Geometry: final body of the model. Coordinates: model frame, mm. A direction names the side the tool comes from. Give positions to 0.01 mm unless a question says otherwise; leave off trailing zeros. Order: outer loops, then holes, each group sorted by start corner. A loop starts at its lowest first (then second) coordinate and runs counter-clockwise, first axis right, second up. Notation, with made-up numbers: (-23, 29) -> (14, 29) arc R11 ccw to (14, 43) -> close; hole circle Ø4 at (-29.5, 28). An arc over 180 degrees is marked (long way). One line per question, with ' | ' between items. Start each with the question number.
(1) Mould query, pull axis X, two halves, no side actions, for faces 1 (the face through (29.083, 8, 11)), 2 (the face through (-38.1, 7, 0)), 3 (the face through (-1, 0, 0)). Classes: +X half, -X half, draft (parallel to the pull), parting line (faces both ways), or undercut.
(2) Section C-C (z = 0). Return loops of the section in (x, y).
(3) Section D-D (z = 19.05). Return loops of the section in (x, y).
(4) Ray query, L1, parallel to Z at x = 0, y = 10; L2, parallel to X at y = 7, z = -19.05; L3, parallel to Z at x = 31.75, y = 4.75. Return the intervals inside material, ascending.
(5) First-contact query: pin 1 Ø3 at (x, z) = (0, -19.05) entering from -Y; pin 2 Ø10 at (x, z) = (-13, -7) entering from +Y. Flat tips, straight axial feed; report the tip coordinate or a pass-through.
(6) Section A-A (x = -31.75). Return loops of the section in (y, z), then the cut area to 3 significant figures.
(7) Section B-B (x = 0). Return loops of the section in (y, z), then the cut area to 3 significant figures.
(8) Set-up query: faces 4 (the face through (33.676, 6.439, -0.607)), 5 (the face through (28.105, 7.879, -7.381)). Return all of +Z, -Z, +X, -X, +Y, -Y with unobstructed straight access to the full face (end or side cutting, diameter ignored); none if empty.
```python
from build123d import *

# Parameters (mm, degrees)
SKETCH1_W              = 76.2
SKETCH1_H              = 50.8
BOSS_EXTRUDE1_DEPTH    = 12.7
SKETCH2_W              = 51.308
SKETCH2_H              = 25.908
CUT_EXTRUDE1_DEPTH     = 9.779
CUT_EXTRUDE2_DEPTH     = 9.779
MIRROR2_COPY_1_DEPTH   = 9.779
F_10_32_TAPPED_HOLE1_D = 4.0386
CHAMFER1_SIZE          = 3.175
FILLET1_R              = 0.508
CHAMFER2_SIZE          = 0.508
F_10_32_TAPPED_HOLE2_D = 4.0386


with BuildPart() as part:
    # Sketch1 → Boss-Extrude1 (new body)
    with BuildSketch(Plane(origin=(0, 0, 0), x_dir=(1, 0, 0), z_dir=(0, 1, 0))):
        Rectangle(SKETCH1_W, SKETCH1_H)
    extrude(amount=BOSS_EXTRUDE1_DEPTH)

    # Sketch2 → Cut-Extrude1 (cut)
    with BuildSketch(Plane(origin=(0, 12.7, 0), x_dir=(1, 0, 0), z_dir=(0, 1, 0))):
        Rectangle(SKETCH2_W, SKETCH2_H)
    extrude(amount=-CUT_EXTRUDE1_DEPTH, mode=Mode.SUBTRACT)

    # Sketch3 → Cut-Extrude2 (cut)
    with BuildSketch(Plane(origin=(0, 12.7, 0), x_dir=(1, 0, 0), z_dir=(0, 1, 0))):
        with BuildLine():
            Line((-22.479, 16.383), (-25.654, 16.383))
            ThreePointArc((-25.654, 16.383), (-28.078669153, 15.378669153), (-29.083, 12.954))
            Line((-29.083, 12.954), (-29.083, 9.779))
            ThreePointArc((-29.083, 9.779), (-26.96622149, 6.611017083), (-23.229330847, 7.354330847))
            Line((-23.229330847, 7.354330847), (-20.054330847, 10.529330847))
            ThreePointArc((-20.054330847, 10.529330847), (-19.311017083, 14.26622149), (-22.479, 16.383))
        make_face()
    cut_extrude2 = extrude(amount=-CUT_EXTRUDE2_DEPTH, mode=Mode.SUBTRACT)

    # Mirror1: Cut-Extrude2 across plane
    add(cut_extrude2.mirror(Plane.XY), mode=Mode.SUBTRACT)

    # Mirror2: Cut-Extrude2 across plane
    add(cut_extrude2.mirror(Plane(origin=(0, 0, 0), x_dir=(0, 0, 1), z_dir=(1, 0, 0))), mode=Mode.SUBTRACT)

    # Mirror2 copy 1 sketch → Mirror2 copy 1 (cut)
    with BuildSketch(Plane(origin=(0, 12.7, 0), x_dir=(-1, 0, 0), z_dir=(0, 1, 0))):
        with BuildLine():
            Line((-22.479, 16.383), (-25.654, 16.383))
            ThreePointArc((-25.654, 16.383), (-28.078669153, 15.378669153), (-29.083, 12.954))
            Line((-29.083, 12.954), (-29.083, 9.779))
            ThreePointArc((-29.083, 9.779), (-26.96622149, 6.611017083), (-23.229330847, 7.354330847))
            Line((-23.229330847, 7.354330847), (-20.054330847, 10.529330847))
            ThreePointArc((-20.054330847, 10.529330847), (-19.311017083, 14.26622149), (-22.479, 16.383))
        make_face()
    extrude(amount=-MIRROR2_COPY_1_DEPTH, mode=Mode.SUBTRACT)

    # #10-32 Tapped Hole1 (through all)
    with Locations(Plane(origin=(0, 12.7, 0), x_dir=(1, 0, 0), z_dir=(0, 1, 0))):
        with Locations((-31.75, 19.05), (31.75, 19.05), (31.75, -19.05), (-31.75, -19.05)):
            Hole(F_10_32_TAPPED_HOLE1_D / 2)

    # Chamfer1
    chamfer1_edges = [part.edges().sort_by_distance(p)[0] for p in [
        (38.1, 6.35, 25.4),
        (-38.1, 6.35, 25.4),
        (-38.1, 6.35, -25.4),
        (38.1, 6.35, -25.4),
    ]]
    chamfer(chamfer1_edges, length=CHAMFER1_SIZE)

    # Fillet1
    fillet1_edges = [part.edges().sort_by_distance(p)[0] for p in [
        (-38.1, 6.35, 22.225),
        (-38.1, 6.35, -22.225),
        (34.925, 6.35, -25.4),
        (-34.925, 6.35, -25.4),
        (38.1, 6.35, 22.225),
        (38.1, 6.35, -22.225),
        (-34.925, 6.35, 25.4),
        (34.925, 6.35, 25.4),
    ]]
    fillet(fillet1_edges, radius=FILLET1_R)

    # Chamfer2
    chamfer2_edges = [part.edges().sort_by_distance(p)[0] for p in [
        (38.1, 0, 0),
        (36.5125, 0, -23.8125),
        (-38.1, 0, 0),
        (-36.5125, 0, -23.8125),
        (0, 0, -25.4),
        (36.5125, 0, 23.8125),
        (0, 0, 25.4),
        (-36.5125, 0, 23.8125),
        (34.908982694, 0, 25.361330803),
        (38.061330803, 0, 22.208982694),
        (-38.061330803, 0, 22.208982694),
        (-34.908982694, 0, 25.361330803),
        (-38.061330803, 0, -22.208982694),
        (-34.908982694, 0, -25.361330803),
        (34.908982694, 0, -25.361330803),
        (38.061330803, 0, -22.208982694),
    ]]
    chamfer(chamfer2_edges, length=CHAMFER2_SIZE)

    # #10-32 Tapped Hole2 (through all)
    with Locations(Plane(origin=(0, 0, 0), x_dir=(-1, 0, 0), z_dir=(0, -1, 0))):
        with Locations((0, 19.05), (0, -19.05), (31.75, 0), (-31.75, 0)):
            Hole(F_10_32_TAPPED_HOLE2_D / 2)


solid = part.part
```
Response:
1) face 1: undercut | face 2: -X half | face 3: draft
2) outline: (-38.1, 0.51) -> (-37.59, 0) -> (-33.77, 0) -> (-33.77, 12.7) -> (-38.1, 12.7) -> close; (-29.73, 0) -> (29.73, 0) -> (29.73, 12.7) -> (25.65, 12.7) -> (25.65, 2.92) -> (-25.65, 2.92) -> (-25.65, 12.7) -> (-29.73, 12.7) -> close; (33.77, 0) -> (37.59, 0) -> (38.1, 0.51) -> (38.1, 12.7) -> (33.77, 12.7) -> close
3) outline: (-38.1, 0.51) -> (-37.59, 0) -> (-33.77, 0) -> (-33.77, 12.7) -> (-38.1, 12.7) -> close; (-29.73, 0) -> (-2.02, 0) -> (-2.02, 12.7) -> (-29.73, 12.7) -> close; (2.02, 0) -> (29.73, 0) -> (29.73, 12.7) -> (2.02, 12.7) -> close; (33.77, 0) -> (37.59, 0) -> (38.1, 0.51) -> (38.1, 12.7) -> (33.77, 12.7) -> close
4) L1: z = -25.4 to -21.07, -17.03 to -12.95, 12.95 to 17.03, 21.07 to 25.4 | L2: x = -38.1 to -33.77, -29.73 to -2.02, 2.02 to 29.73, 33.77 to 38.1 | L3: z = -25.4 to -21.07, -17.03 to -2.02, 2.02 to 17.03, 21.07 to 25.4
5) pin 1: passes through | pin 2: stops at y = 2.92
6) outline: (0, -24.89) -> (0.51, -25.4) -> (12.7, -25.4) -> (12.7, -21.07) -> (0, -21.07) -> close; (0, -17.03) -> (12.7, -17.03) -> (12.7, -2.02) -> (0, -2.02) -> close; (0, 2.02) -> (12.7, 2.02) -> (12.7, 17.03) -> (0, 17.03) -> close; (0, 21.07) -> (12.7, 21.07) -> (12.7, 25.4) -> (0.51, 25.4) -> (0, 24.89) -> close | area: 491 mm^2
7) outline: (0, -24.89) -> (0.51, -25.4) -> (12.7, -25.4) -> (12.7, -21.07) -> (0, -21.07) -> close; (0, -17.03) -> (12.7, -17.03) -> (12.7, -12.95) -> (2.92, -12.95) -> (2.92, 12.95) -> (12.7, 12.95) -> (12.7, 17.03) -> (0, 17.03) -> close; (0, 21.07) -> (12.7, 21.07) -> (12.7, 25.4) -> (0.51, 25.4) -> (0, 24.89) -> close | area: 289 mm^2
8) face 4: +Y, -Y | face 5: +Y
